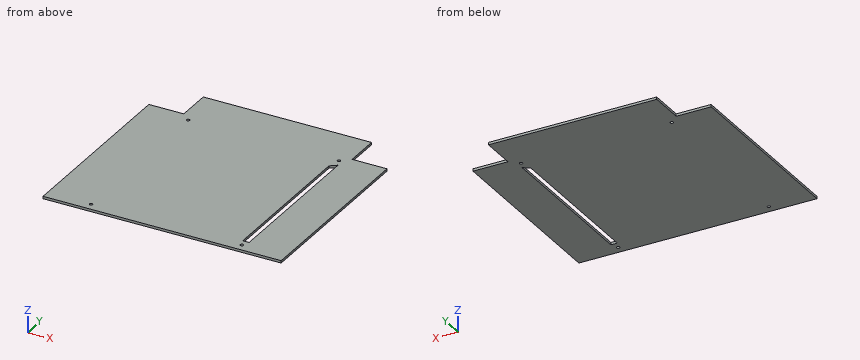
from build123d import *

# Parameters (mm, degrees)
SKETCH1_R           = 2
BOSS_EXTRUDE1_DEPTH = 3


with BuildPart() as part:
    # Sketch1 → Boss-Extrude1 (new body)
    with BuildSketch(Plane.XY):
        Polygon((-150, -119.5), (150, -119.5), (150, 119.5), (106, 119.5), (106, 163.5), (-106, 163.5), (-106, 119.5), (-150, 119.5), align=None)
        with Locations((-95, -109.5)):
            Circle(SKETCH1_R, mode=Mode.SUBTRACT)
        with Locations((95, -109.5)):
            Circle(SKETCH1_R, mode=Mode.SUBTRACT)
        Polygon((91, 94.126666667), (99, 100.5), (99, -100.5), (91, -100.5), align=None, mode=Mode.SUBTRACT)
        with Locations((-95, 109.5)):
            Circle(SKETCH1_R, mode=Mode.SUBTRACT)
        with Locations((95, 109.5)):
            Circle(SKETCH1_R, mode=Mode.SUBTRACT)
    extrude(amount=BOSS_EXTRUDE1_DEPTH)


solid = part.part
Verification items for the finished model (mm, model axes). Give positions to 0.01 mm unless a question says otherwise; leave off trailing zeros. Loops run counter-clockwise (first coordinate to the right, second up) from the corner with the lowest first, then second, coordinate; pieces in that order, holes last. Notation, with made-up numbers: (0, -39) - (31, -39) arc R19 cw to (31, -12) - close; hole circle Ø4 at (44.5, 85). An arc over 180 degrees is marked (long way). Write item = value, one per line. Start each with the question number.
Q1. Thickness scan on line 1 (Y direction, x = -95, z = 1.8); line 2 (X direction, y = -83, z = 0.6); line 3 (Y direction, x = 95, z = 1.35). Record the ranges inside material, lowest first.
Q2. Depth check by flat-ended pin: P1, Ø1.5, axis at x = -137.5, z = 1.5, coming from the +Y side; P2, Ø8, axis at x = 42, y = 71, coming from the -Z side. Enter the tip coordinate at first touch or a pass-through.
Q3. Cross-section at A-A, the plane y = 19. Enter the section's corners in (x, z), and give its area (3 significant figures).
Q4. Cross-section at B-B, the plane z = 1.25. Enter the section's corners in (x, y).
Answer key:
q1.line_1 = -119.5 to -111.5, -107.5 to 107.5, 111.5 to 163.5
q1.line_2 = -150 to 91, 99 to 150
q1.line_3 = -119.5 to -111.5, -107.5 to -100.5, 97.31 to 107.5, 111.5 to 163.5
q2.P1 = 119.5
q2.P2 = 0
q3.outline = (-150, 0) - (91, 0) - (91, 3) - (-150, 3) - close; (99, 0) - (150, 0) - (150, 3) - (99, 3) - close
q3.area = 876 mm^2
q4.outline = (-150, -119.5) - (150, -119.5) - (150, 119.5) - (106, 119.5) - (106, 163.5) - (-106, 163.5) - (-106, 119.5) - (-150, 119.5) - close; hole circle Ø4 at (-95, -109.5); hole circle Ø4 at (-95, 109.5); hole (91, -100.5) - (99, -100.5) - (99, 100.5) - (91, 94.13) - close; hole circle Ø4 at (95, -109.5); hole circle Ø4 at (95, 109.5)
